Work out the finished part from the listing and answer in its coordinate system (mm). Face numbers are marked on the shaded views. A direction names the side the tool comes from. Give positions to 0.01 mm unless a question says otherwise; leave off trailing zeros. Loops run counter-clockwise (first coordinate to the right, second up) from the corner with the lowest first, then second, coordinate; pieces in that order, holes last. Notation, with made-up numbers: M 65.25,-17 L 75.25,-17 A20 cw 75.25,18 Z; hole C -23.75,55.5 d3. An arc over 180 degrees is marked long. Use a Markdown table: item, result.
```python
from build123d import *

# Parameters (mm, degrees)
BOSS_EXTRUDE2_DEPTH = 6.5
CUT_EXTRUDE1_START  = 44.888544
SKETCH3_R           = 2
CUT_EXTRUDE1_DEPTH  = 9.111456


with BuildPart() as part:
    # Sketch1 → Boss-Extrude2 (new body, symmetric)
    with BuildSketch(Plane.XY):
        with BuildLine():
            Line((-13.5, 0), (-23, 0))
            Line((-23, 0), (-23, 27))
            ThreePointArc((-23, 27), (-18.183096546, 41.084566021), (-5.75, 49.269654241))
            ThreePointArc((-5.75, 49.269654241), (-5.209430585, 49.625527642), (-5, 50.237900077))
            Line((-5, 50.237900077), (-5, 51))
            ThreePointArc((-5, 51), (-4.121320344, 53.121320344), (-2, 54))
            Line((-2, 54), (2, 54))
            ThreePointArc((2, 54), (4.121320344, 53.121320344), (5, 51))
            Line((5, 51), (5, 50.237900077))
            ThreePointArc((5, 50.237900077), (5.209430585, 49.625527642), (5.75, 49.269654241))
            ThreePointArc((5.75, 49.269654241), (18.183096546, 41.084566021), (23, 27))
            Line((23, 27), (23, 0))
            Line((23, 0), (13.5, 0))
            Line((13.5, 0), (13.5, 3))
            Line((13.5, 3), (18, 3))
            Line((18, 3), (18, 27))
            ThreePointArc((18, 27), (12.727922061, 39.727922061), (0, 45))
            ThreePointArc((0, 45), (-12.727922061, 39.727922061), (-18, 27))
            Line((-18, 27), (-18, 3))
            Line((-18, 3), (-13.5, 3))
            Line((-13.5, 3), (-13.5, 0))
        make_face()
    extrude(amount=BOSS_EXTRUDE2_DEPTH, both=True)

    # Sketch3 → Cut-Extrude1 (cut)
    with BuildSketch(Plane(origin=(0, 0, 0), x_dir=(1, 0, 0), z_dir=(0, 1, 0)).offset(CUT_EXTRUDE1_START)):
        with Locations((0, -0.5)):
            Circle(SKETCH3_R)
    extrude(amount=CUT_EXTRUDE1_DEPTH, mode=Mode.SUBTRACT)


solid = part.part
```
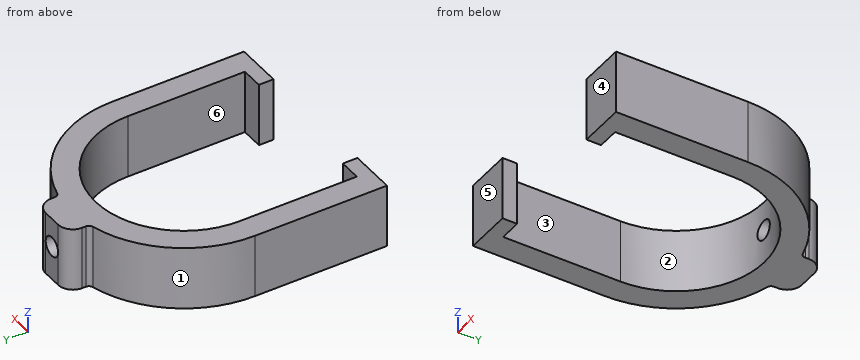
(1) Which of the six approach directions +Z, -Z, +X, -X, +Y, -Y give full straight-line access (tool end or side, diameter ignored) to the marked faces 5 and 6?
Entries:
| item | result |
|---|---|
| face 5 | +Z, -Z, +X, -X, -Y |
| face 6 | +Z, -Z |
(2) Given P1, Ø4, axis at y = 31, z = -0.5, coming from the +X side; P2, Ø3.5, axis at x = 15.5, z = -2, coming from the +Y side; P3, Ø2, axis at x = -14.5, z = -1.5, coming from the +Y side, each flat-ended and moving along its own axis, determine where each tip first touches the part or whether it passes through.
Entries:
| item | result |
|---|---|
| P1 | stops at x = 22.91 |
| P2 | stops at y = 45.44 |
| P3 | stops at y = 45.62 |
(3) Consider probe 1 along X at (y, z) = (17.5, 6); probe 2 along Z at (x, y) = (0, 50.25); probe 3 along X at (y, z) = (50.75, 0.5). Determine where each line is inside the solid, lowest interval first. Write a range as [from, to].
Entries:
| item | result |
|---|---|
| probe 1 | x = [-23, -18], [18, 23] |
| probe 2 | z = [-6.5, -1.5], [2.5, 6.5] |
| probe 3 | x = [-5, -2], [2, 5] |
(4) A cutting plane is placed at A-A (x = 0). Write down the section's boundary in (y, z).
Entries:
| item | result |
|---|---|
| outline | M 45,-6.5 L 54,-6.5 L 54,-1.5 L 45,-1.5 Z; M 45,2.5 L 54,2.5 L 54,6.5 L 45,6.5 Z |
(5) A cutting plane is placed at D-D (x = -11.5). Write down the section's boundary in (y, z).
Entries:
| item | result |
|---|---|
| outline | M 40.85,-6.5 L 46.92,-6.5 L 46.92,6.5 L 40.85,6.5 Z |
(6) A cutting plane is placed at B-B (z = 5). Write down the section's boundary in (x, y).
Entries:
| item | result |
|---|---|
| outline | M -23,0 L -13.5,0 L -13.5,3 L -18,3 L -18,27 A18 cw 18,27 L 18,3 L 13.5,3 L 13.5,0 L 23,0 L 23,27 A23 ccw 5.75,49.27 A1 cw 5,50.24 L 5,51 A3 ccw 2,54 L -2,54 A3 ccw -5,51 L -5,50.24 A1 cw -5.75,49.27 A23 ccw -23,27 Z |
(7) The mould has two halves that part along Y. Classify the marked faces 1, 2, 3 and 4: released by +Y, released by -Y, zero draft, split by the parting line, or undercut.
Entries:
| item | result |
|---|---|
| face 1 | released by +Y |
| face 2 | undercut |
| face 3 | undercut |
| face 4 | released by -Y |
(8) A cutting plane is placed at C-C (y = 37). Write down the section's boundary in (x, z).
Entries:
| item | result |
|---|---|
| outline | M -20.71,-6.5 L -14.97,-6.5 L -14.97,6.5 L -20.71,6.5 Z; M 14.97,-6.5 L 20.71,-6.5 L 20.71,6.5 L 14.97,6.5 Z |
